from build123d import *

# Parameters (mm, degrees)
SKETCH1_R           = 3.5
BOSS_EXTRUDE1_DEPTH = 13
CHAMFER1_SIZE       = 2


with BuildPart() as part:
    # Sketch1 → Boss-Extrude1 (new body)
    with BuildSketch(Plane.XY):
        with BuildLine():
            ThreePointArc((24.387496797, 5.5), (17.858383307, 17.495089187), (6, 24.269322199))
            Line((6, 24.269322199), (6, 12))
            ThreePointArc((6, 12), (0, 6), (-6, 12))
            Line((-6, 12), (-6, 24.269322199))
            ThreePointArc((-6, 24.269322199), (-17.494151854, 17.859301524), (-24.140215409, 6.5))
            Line((-24.140215409, 6.5), (-12, 6.5))
            ThreePointArc((-12, 6.5), (-5.5, 0), (-12, -6.5))
            Line((-12, -6.5), (-24.140215409, -6.5))
            ThreePointArc((-24.140215409, -6.5), (-17.124313764, -18.214221864), (-5, -24.494897428))
            Line((-5, -24.494897428), (-5, -12))
            ThreePointArc((-5, -12), (0, -7), (5, -12))
            Line((5, -12), (5, -24.494897428))
            ThreePointArc((5, -24.494897428), (17.49593593, -17.85755375), (24.387496797, -5.5))
            Line((24.387496797, -5.5), (12, -5.5))
            ThreePointArc((12, -5.5), (6.5, 0), (12, 5.5))
            Line((12, 5.5), (24.387496797, 5.5))
        make_face()
        with Locations(Location((0, 0, 0), (0, 0, 180))):
            Circle(SKETCH1_R, mode=Mode.SUBTRACT)
    extrude(amount=BOSS_EXTRUDE1_DEPTH)

    # Chamfer1
    chamfer1_edges = [part.edges().sort_by_distance(p)[0] for p in [
        (17.49593593, -17.85755375, 13),
        (17.858383307, 17.495089187, 13),
        (-17.494151854, 17.859301524, 13),
        (-17.124313764, -18.214221864, 13),
    ]]
    chamfer(chamfer1_edges, length=CHAMFER1_SIZE)


solid = part.part
CAD build for the part. Positions are in the model's coordinates, mm. A direction names the side the tool comes from. Round coordinates to 2 decimals unless told otherwise and drop trailing zeros. Loops run counter-clockwise (first coordinate to the right, second up) from the corner with the lowest first, then second, coordinate; pieces in that order, holes last.
(1) Cut at B-B (z = 2.75). Give the cut face in (x, y).
(2) Two-plate mould, pull along X, no slides. Class faces 1 (the flat face through (-18, 6.5, 6)), 2 (the cylindrical face through (6.5, -0.1, 6.4)), 3 (the cylindrical face through (0, -7, 6)), 4 (the cylindrical face through (-3.233, 1.341, 6.409)): +X half, -X half, draft (parallel to the pull), parting line (faces both ways), or undercut.
(3) Cut at C-C (z = 12.25). Give the cut face in (x, y), plus the area to 3 significant figures.
(4) Which spindle directions (+Z, -Z, +X, -X, +Y, -Y) get a long thin tool onto all of the face, cutting with end or side? Do faces 5 (the flat face through (-6, 18, 6)), 6 (the conical face through (-16.348, 16.94, 12.458)), 7 (the flat face through (5, -18, 6)), 8 (the cylindrical face through (-17.36, 17.99, 5.42)), 9 (the flat face through (18, 5.5, 6)). Say none if no direction does.
(5) Wall check: line 1 along Y through (x, z) = (0, 4.25); line 2 along X through (y, z) = (18.5, 8.25); line 3 along Y through (x, z) = (22.5, 7.5). Give the ranges that are in metal, low to high.
(6) Drop flat-ended pins along their axis: pin 1 (4 mm diameter, centred on x = 8, z = 8.5, fed in from -Y); pin 2 (6 mm diameter, centred on x = -17.5, z = 9.5, fed in from -Y); pin 3 (6 mm diameter, centred on x = -15.5, z = 9, fed in from +Y); pin 4 (4 mm diameter, centred on x = 0, y = 0, fed in from +Z). Give the stop position or say it passes through.
(7) Cut at A-A (x = 0). Give the cut face in (y, z), plus the area to 3 significant figures.
Findings below:
1. outline: (-24.14, -6.5) arc R25 ccw to (-5, -24.49) - (-5, -12) arc R5 cw to (5, -12) - (5, -24.49) arc R25 ccw to (24.39, -5.5) - (12, -5.5) arc R5.5 cw to (12, 5.5) - (24.39, 5.5) arc R25 ccw to (6, 24.27) - (6, 12) arc R6 cw to (-6, 12) - (-6, 24.27) arc R25 ccw to (-24.14, 6.5) - (-12, 6.5) arc R6.5 cw to (-12, -6.5) - close; hole circle Ø7 at (0, 0)
2. face 1: draft
2. face 2: +X half
2. face 3: undercut
2. face 4: undercut
3. outline: (-22.84, -6.5) arc R23.75 ccw to (-5, -23.22) - (-5, -12) arc R5 cw to (5, -12) - (5, -23.22) arc R23.75 ccw to (23.1, -5.5) - (12, -5.5) arc R5.5 cw to (12, 5.5) - (23.1, 5.5) arc R23.75 ccw to (6, 22.98) - (6, 12) arc R6 cw to (-6, 12) - (-6, 22.98) arc R23.75 ccw to (-22.84, 6.5) - (-12, 6.5) arc R6.5 cw to (-12, -6.5) - close; hole circle Ø7 at (0, 0)
3. area: 994 mm2
4. face 5: +Z, -Z, +Y
4. face 6: +Z, -X, +Y
4. face 7: +Z, -Z, -Y
4. face 8: +Z, -Z, -X, +Y
4. face 9: +Z, -Z, +X
5. line 1: y = -7 to -3.5, 3.5 to 6
5. line 2: x = -16.82 to -6, 6 to 16.82
5. line 3: y = -10.9 to -5.5, 5.5 to 10.9
6. pin 1: stops at y = -24.27
6. pin 2: stops at y = -20.37
6. pin 3: stops at y = 21.65
6. pin 4: passes through
7. outline: (-7, 0) - (-3.5, 0) - (-3.5, 13) - (-7, 13) - close; (3.5, 0) - (6, 0) - (6, 13) - (3.5, 13) - close
7. area: 78.0 mm2
